Can you work these out from the model? Positions are in its coordinate system, mm. Coordinates: 2 decimals unless noted, no trailing zeros. Order: outer loops, then holes, each group sorted by start corner. A loop starts at its lowest first (then second) coordinate and runs counter-clockwise, first axis right, second up. Notation, with made-up numbers: (-9, 82.25) -> (29, 82.25) arc R26 cw to (29, 113.25) -> close; hole circle Ø1 at (32, -33.5). An arc over 180 degrees is marked (long way). Return JSON: item names as keys, results as strings. Group by question number.
1) If we section it at A-A, the plane x = 0: Please give me the cut outline in (y, z).
2) If we section it at C-C, the plane z = 15: Please give me the cut outline in (x, y), then the cut area to 3 significant figures.
3) If we section it at B-B, the plane y = 0: Please give me the cut outline in (x, z), then the cut area to 3 significant figures.
4) Thinking about a two-plate mould opening in Y: for faces 1 (the flat face through (5, 0, 11)), 2 (the cylindrical face through (1.5, 0.07, 10.85)), 3 (the flat face through (0, 3, 11)), which applies, +Y half, -Y half, draft (parallel to the pull), parting line (faces both ways), or undercut?
5) For pin 1 (1.8 mm diameter, centred on x = 0, y = 0, fed in from +Z), with a flat end and sliding along its axis, tell me the tip position at first contact or that it passes through.
6) If I drill on probe 1 along Y at (x, z) = (0, 16.25); probe 2 along Y at (x, z) = (-1, 3); probe 3 along X at (y, z) = (-1.25, 4.75), over which ranges is the centre line in solid material (lowest first)? Write a range as from..to.
from build123d import *

# Parameters (mm, degrees)
SKETCH_1_W          = 10
SKETCH_1_H          = 6
EXTRUDE_1_DEPTH     = 22
SKETCH_3_R          = 1.5
CUT_EXTRUDE_1_DEPTH = 23.759613353
CHAMFER_1_SIZE      = 0.3


with BuildPart() as part:
    # 草图1 → 凸台-拉伸1 (new body)
    with BuildSketch(Plane.XY):
        Rectangle(SKETCH_1_W, SKETCH_1_H)
    extrude(amount=EXTRUDE_1_DEPTH)

    # 草图3 → 切除-拉伸1 (cut, through all)
    with BuildSketch(Plane(origin=(0, 0, 0), x_dir=(-1, 0, 0), z_dir=(0, 0, -1))):
        Circle(SKETCH_3_R)
    extrude(amount=-CUT_EXTRUDE_1_DEPTH, mode=Mode.SUBTRACT)

    # 倒角1
    chamfer_1_edges = [part.edges().sort_by_distance(p)[0] for p in [
        (-5, 0, 22),
        (1.5, 0, 22),
        (1.5, 0, 0),
        (0, -3, 22),
        (5, 0, 22),
        (0, -3, 0),
        (-5, 0, 0),
        (0, 3, 0),
        (5, 0, 0),
        (5, -3, 11),
        (-5, -3, 11),
        (-5, 3, 11),
        (5, 3, 11),
        (0, 3, 22),
    ]]
    chamfer(chamfer_1_edges, length=CHAMFER_1_SIZE)


solid = part.part
Result sheet:
{
 "1": {"outline": "(-3, 0.3) -> (-2.7, 0) -> (-1.8, 0) -> (-1.5, 0.3) -> (-1.5, 21.7) -> (-1.8, 22) -> (-2.7, 22) -> (-3, 21.7) -> close; (1.5, 0.3) -> (1.8, 0) -> (2.7, 0) -> (3, 0.3) -> (3, 21.7) -> (2.7, 22) -> (1.8, 22) -> (1.5, 21.7) -> close"},
 "2": {"outline": "(-5, -2.7) -> (-4.7, -3) -> (4.7, -3) -> (5, -2.7) -> (5, 2.7) -> (4.7, 3) -> (-4.7, 3) -> (-5, 2.7) -> close; hole circle Ø3 at (0, 0)", "area": "52.8 mm2"},
 "3": {"outline": "(-5, 0.3) -> (-4.7, 0) -> (-1.8, 0) -> (-1.5, 0.3) -> (-1.5, 21.7) -> (-1.8, 22) -> (-4.7, 22) -> (-5, 21.7) -> close; (1.5, 0.3) -> (1.8, 0) -> (4.7, 0) -> (5, 0.3) -> (5, 21.7) -> (4.7, 22) -> (1.8, 22) -> (1.5, 21.7) -> close", "area": "154 mm2"},
 "4": {"face 1": "draft", "face 2": "undercut", "face 3": "+Y half"},
 "5": {"pin 1": "passes through"},
 "6": {"probe 1": "y = -3..-1.5, 1.5..3", "probe 2": "y = -3..-1.12, 1.12..3", "probe 3": "x = -5..-0.83, 0.83..5"}
}
